Read the model definition and answer for the solid it produces. Units are mm, in the model's axes. A direction names the side the tool comes from. Coordinates: 2 decimals unless noted, no trailing zeros. Order: outer loops, then holes, each group sorted by start corner. A loop starts at its lowest first (then second) coordinate and runs counter-clockwise, first axis right, second up. Notation, with made-up numbers: (5.5, -3.5) -> (33.5, -3.5) arc R18 cw to (33.5, 22.5) -> close; hole circle Ø8 at (32, 78.5). An arc over 180 degrees is marked (long way). Use CSV: the item, a comma, the result in double quotes.
Autodesk Inventor part; units mm, degrees
ref_plane "Plano de trabajo1" through (75, 0, 0) normal (1, 0, 0) x (0, 0, -1)
ref_plane "Plano de trabajo2" through (150, 25, 68) normal (0, 0, 1) x (1, 0, 0)
ref_plane "Plano de trabajo3" through (75, 0, 0) normal (1, 0, 0) x (0, 0, -1)
sketch "Boceto1" plane through (0, 0, 0) normal (0, 0, 1) x (1, 0, 0)
  line L0 (0, 0) -> (150, 0)
  line L1 (150, 0) -> (150, 150)
  line L2 (150, 150) -> (0, 150)
  line L3 (0, 150) -> (0, 0)
  line L4 (5, 145) -> (145, 145)
  line L5 (145, 145) -> (145, 5)
  line L6 (145, 5) -> (5, 5)
  line L7 (5, 5) -> (5, 145)
  dimension "d0" = 150
  dimension "d1" = 150
  dimension "d2" = 5
extrude "Extrusión1" add sketch "Boceto1" along normal blind 150
sketch "Boceto2" plane through (150, 0, 0) normal (1, 0, 0) x (0, 0, -1)
  line L0 (-150, 0) -> (-150, 150)
  line L1 (-150, 75) -> (-190, 75) construction
  line L2 (-190, 75) -> (-150, 150)
  line L3 (0, 0) -> (-150, 0) construction
  line L4 (-150, 0) -> (-190, 75)
  dimension "d5" = 40
extrude "Extrusión2" add sketch "Boceto2" against normal blind 5
ref_plane "Plano de trabajo1" through (75, 0, 0) normal (1, 0, 0) x (0, 0, -1)
mirror "Simetría1" about plane through (75, 0, 0) normal (1, 0, 0) of "Extrusión2"
sketch "Boceto3" plane through (0, 150, 0) normal (0, 1, 0) x (1, 0, 0)
  line L0 (105, -60) -> (45, -60)
  line L1 (45, -60) -> (45, -95)
  line L2 (60, -110) -> (90, -110)
  line L3 (105, -95) -> (105, -60)
  line L4 (150, 0) -> (0, 0)
  line L5 (145, -150) -> (5, -150)
  arc A0 (90, -110) -> (105, -95) centre (90, -95) ccw
  arc A1 (45, -95) -> (60, -110) centre (60, -95) ccw
  point P0 (45, -110)
  point P1 (105, -110)
  point P2 (75, -60)
  point P3 (75, 0)
  dimension "d8" = 60
  dimension "d9" = 50
  dimension "d10" = 40
  dimension "d11" = 15
extrude "Extrusión3" cut sketch "Boceto3" against normal through all
sketch "Boceto4" plane through (150, 0, 0) normal (1, 0, 0) x (0, 0, -1)
  line L0 (-13, 20) -> (-123, 20)
  line L1 (-128, 25) -> (-128, 75)
  line L2 (-123, 80) -> (-13, 80)
  line L3 (-8, 75) -> (-8, 25)
  line L4 (0, 0) -> (0, 150)
  line L5 (0, 0) -> (-150, 0)
  arc A0 (-123, 80) -> (-128, 75) centre (-123, 75) ccw
  arc A1 (-8, 75) -> (-13, 80) centre (-13, 75) ccw
  arc A2 (-13, 20) -> (-8, 25) centre (-13, 25) ccw
  arc A3 (-128, 25) -> (-123, 20) centre (-123, 25) ccw
  point P0 (-128, 80)
  point P1 (-128, 20)
  point P2 (-8, 80)
  dimension "d14" = 120
  dimension "d15" = 60
  dimension "d16" = 8
  dimension "d17" = 20
  dimension "d18" = 5
extrude "Extrusión4" cut sketch "Boceto4" against normal up to surface (5 mm away)
sketch "Boceto5" plane through (0, 0, 0) normal (-1, 0, 0) x (0, 0, 1)
  line L0 (65, 125) -> (115, 125)
  line L1 (120, 120) -> (120, 30)
  line L2 (115, 25) -> (65, 25)
  line L3 (60, 30) -> (60, 120)
  line L4 (0, 150) -> (0, 0)
  arc A0 (120, 120) -> (115, 125) centre (115, 120) ccw
  arc A1 (115, 25) -> (120, 30) centre (115, 30) ccw
  arc A2 (65, 125) -> (60, 120) centre (65, 120) ccw
  arc A3 (60, 30) -> (65, 25) centre (65, 30) ccw
  point P0 (60, 150)
  point P1 (120, 25)
  point P2 (120, 125)
  point P3 (60, 25)
  point P4 (60, 75)
  point P5 (0, 75)
  dimension "d21" = 60
  dimension "d22" = 100
  dimension "d23" = 60
  dimension "d24" = 5
extrude "Extrusión5" cut sketch "Boceto5" against normal blind 10
sketch "Boceto6" plane through (150, 0, 0) normal (1, 0, 0) x (0, 0, -1)
  line L0 (-190, 75) -> (-150, 0)
  line L1 (-150, 150) -> (-190, 75)
  line L2 (-154.4118, 152.3529) -> (-195.6667, 75)
  line L3 (-195.6667, 75) -> (-154.4118, -2.3529)
  line L4 (-154.4118, 152.3529) -> (-144.4118, 152.3529)
  line L5 (-144.4118, 152.3529) -> (-144.4118, 150)
  line L6 (-154.4118, -2.3529) -> (-144.4118, -2.3529)
  line L7 (-144.4118, -2.3529) -> (-144.4118, 0)
  line L8 (0, 0) -> (-150, 0)
  line L9 (0, 150) -> (-150, 150)
  dimension "d27" = 5
  dimension "d28" = 10
extrude "Extrusión6" add sketch "Boceto6" along normal blind 10 and the other way blind 160
fillet "Empalme1" radius 5 3 edges at (75, 152.3529, 154.4118) (75, 75, 195.6667) (75, -2.3529, 154.4118)
sketch "Boceto7" plane through (150, 25, 8) normal (0, 0, 1) x (1, 0, 0)
  circle A0 centre (-2.5, 2.5) radius 1.25
  line L0 (0, 50) -> (0, 0)
  line L1 (0, 0) -> (-5, 0)
  point P0 (-150, -25)
  point P1 (-2.5, 0)
  dimension "d34" = 2.5
  dimension "d35" = 2.5
  dimension "d36" = 2.5
extrude "Extrusión7" cut sketch "Boceto7" against normal blind 3
ref_plane "Plano de trabajo2" through (150, 25, 68) normal (0, 0, 1) x (1, 0, 0)
mirror "Simetría2" about plane through (150, 25, 68) normal (0, 0, 1) of "Extrusión7"
sketch "Boceto8" plane through (160, 0, 0) normal (1, 0, 0) x (0, 0, -1)
  arc A0 (-155.8235, 0.2941) -> (-151.4118, -2.3529) centre (-151.4118, 2.6471) ccw
  line L0 (-151.4118, -2.3529) -> (-144.4118, -2.3529)
  line L1 (-144.4118, -2.3529) -> (-144.4118, 0)
  line L2 (-144.4118, 0) -> (-150, 0)
  line L3 (-150, 0) -> (-190, 75)
  line L4 (-190, 75) -> (-150, 150)
  line L5 (-150, 150) -> (-144.4118, 150)
  line L6 (-144.4118, 150) -> (-144.4118, 152.3529)
  line L7 (-144.4118, 152.3529) -> (-151.4118, 152.3529)
  arc A1 (-151.4118, 152.3529) -> (-155.8235, 149.7059) centre (-151.4118, 147.3529) ccw
  line L8 (-155.8235, 149.7059) -> (-194.4118, 77.3529)
  arc A2 (-194.4118, 77.3529) -> (-194.4118, 72.6471) centre (-190, 75) ccw
  line L9 (-194.4118, 72.6471) -> (-155.8235, 0.2941)
  point P0 (0, 0)
extrude "Extrusión8" cut sketch "Boceto8" against normal through all
sketch "Boceto9" plane through (145, 0, 150) normal (0, -0.4705882, 0.8823529) x (1, 0, 0)
  circle A0 centre (2.5, 2.5) radius 1.5
  line L0 (5, 85) -> (5, 0)
  line L1 (5, 0) -> (0, 0)
  point P0 (-145, -70.5882)
  dimension "d41" = 3
  dimension "d42" = 2.5
  dimension "d43" = 2.5
extrude "Extrusión9" cut sketch "Boceto9" against normal blind 5
ref_plane "Plano de trabajo3" through (75, 0, 0) normal (1, 0, 0) x (0, 0, -1)
ref_plane "Plano de trabajo4" through (0, 75, 0) normal (0, -1, 0) x (1, 0, 0)
mirror "Simetría3" about plane through (75, 0, 0) normal (1, 0, 0) of "Extrusión9"
mirror "Simetría4" about plane through (0, 75, 0) normal (0, -1, 0) of "Extrusión8", "Extrusión9", "Simetría3"
sketch "Boceto10" plane through (150, 0, 0) normal (1, 0, 0) x (0, 0, -1)
  arc A0 (-13, 20) -> (-8, 25) centre (-13, 25) ccw
  line L0 (-13, 20) -> (-123, 20)
  arc A1 (-128, 25) -> (-123, 20) centre (-123, 25) ccw
  line L1 (-128, 25) -> (-128, 75)
  arc A2 (-123, 80) -> (-128, 75) centre (-123, 75) ccw
  line L2 (-123, 80) -> (-13, 80)
  arc A3 (-8, 75) -> (-13, 80) centre (-13, 75) ccw
  line L3 (-8, 75) -> (-8, 25)
  line L4 (0, 0) -> (0, 150)
  line L5 (0, 150) -> (-150, 150)
  line L6 (-150, 150) -> (-190, 75)
  line L7 (-190, 75) -> (-150, 0)
  line L8 (0, 0) -> (-150, 0)
  point P0 (0, 0)
extrude "Extrusión10" cut sketch "Boceto10" against normal up to surface (145 mm away) contours L0 A1 L1 A2 L2 A3 L3 A0 | L8 L7 L6 L5 L4
sketch "Boceto11" plane through (5, 0, 0) normal (1, 0, 0) x (0, 0, -1)
  circle A0 centre (-147.5, 2.5) radius 1.5
  line L0 (0, 0) -> (-150, 0)
  line L1 (-190, 75) -> (-150, 0) construction
  line L2 (-190, 75) -> (75.3721, 75) construction
  line L3 (-75, 153.8029) -> (-75, -92.275) construction
  circle A1 centre (-147.5, 147.5) radius 1.5
  circle A2 centre (-2.5, 2.5) radius 1.5
  circle A3 centre (-2.5, 147.5) radius 1.5
  dimension "d48" = 3
  dimension "d49" = 2.5
  dimension "d50" = 2.5
extrude "Extrusión11" add sketch "Boceto11" along normal blind 5
properties part number "CasaJugueteAPM" material "Plástico ABS"
Item 1: Straight lines are drawn through the part: line 1 along Y through (x, z) = (4.5, 65); line 2 along Y through (x, z) = (2, 148); line 3 along X through (y, z) = (11.5, 46). For each, find the intervals that lie inside material, in ascending order.
Return value:
line 1,"y = 0 to 25, 125 to 150"
line 2,"y = 0 to 2.3, 5.5 to 144.5, 147.7 to 150"
line 3,"x = 0 to 5"
Item 2: Find section C-C, the plane z = 63. Give the vertices of the cut face in (x, y), then the cut area to 3 significant figures.
Return value:
outline,"(0, 0) -> (5, 0) -> (5, 25.42) -> (0, 25.42) -> close; (0, 124.58) -> (5, 124.58) -> (5, 150) -> (0, 150) -> close"
area,"254 mm^2"
Item 3: A tool of negligible diameter and unlimited length cuts with its end or side. For faces 4 (the flat face through (2, 74, 60)), 5 (the cylindrical face through (1.114, 147.141, 148.73)), from which of +Z, -Z, +X, -X, +Y, -Y can it reach the whole face along a straight path? Write none if from no direction.
Return value:
face 4,"+X, -X"
face 5,"none"
Item 4: Each of these flat-tipped pins is pushed along its axis until it touches: P1, Ø1.5, axis at x = 5.5, y = 103, coming from the +Z side; P2, Ø2, axis at y = 103.5, z = 45, coming from the +X side; P3, Ø5.5, axis at x = 3.5, y = 86.5, coming from the +Z side. Where does it stop, or does it pass through?
Return value:
P1,"stops at z = 175.36"
P2,"stops at x = 5"
P3,"stops at z = 185.33"
Item 5: The mould has two halves that part along X. Classify faces 1 (the cylindrical face through (2, 124, 62)), 2 (the cylindrical face through (1.114, 3.873, 149.271)), 3 (the flat face through (0, 76, 51)): +X half, -X half, draft (parallel to the pull), parting line (faces both ways), or undercut.
Return value:
face 1,"draft"
face 2,"undercut"
face 3,"-X half"
Item 6: Find section B-B, the plane x = 8. Give the vertices of the cut face in (y, z), then the cut area to 3 significant figures.
Return value:
outline,"circle Ø3 at (2.5, 2.5); circle Ø3 at (2.5, 147.5); circle Ø3 at (147.5, 2.5); circle Ø3 at (147.5, 147.5)"
area,"28.3 mm^2"
Item 7: Find section D-D, the plane z = 176. Give the vertices of the cut face in (x, y).
Return value:
outline,"(0, 48.75) -> (5, 48.75) -> (5, 101.25) -> (0, 101.25) -> close"
Item 8: Find section A-A, the plane y = 43.5. Give the vertices of the cut face in (x, z).
Return value:
outline,"(0, 0) -> (5, 0) -> (5, 60) -> (0, 60) -> close; (0, 120) -> (5, 120) -> (5, 173.2) -> (0, 173.2) -> close"
